```python
from build123d import *

# Parameters (mm, degrees)
SKETCH_W        = 100
SKETCH_H        = 84
PAD_DEPTH       = 10
SKETCH001_R     = 2.1
POCKET_DEPTH    = 10
SKETCH002_R     = 2.1
POCKET001_DEPTH = 10
SKETCH003_R     = 4
POCKET002_DEPTH = 4
SKETCH004_R     = 4
POCKET003_DEPTH = 4
SKETCH005_R     = 3.1
POCKET004_DEPTH = 10
SKETCH006_R     = 4.8
POCKET005_DEPTH = 5.2


with BuildPart() as part:
    # Sketch → Pad (new body)
    with BuildSketch(Plane.XY):
        with Locations((50, 42)):
            Rectangle(SKETCH_W, SKETCH_H)
    extrude(amount=PAD_DEPTH)

    # Sketch001 (on Face6 of Pad) → Pocket (cut)
    with BuildSketch(Plane.XY.offset(10)):
        with Locations((5, 6)):
            Circle(SKETCH001_R)
        with Locations((29, 6)):
            Circle(SKETCH001_R)
        with Locations((71, 6)):
            Circle(SKETCH001_R)
        with Locations((95, 6)):
            Circle(SKETCH001_R)
        with Locations((5, 24)):
            Circle(SKETCH001_R)
        with Locations((29, 24)):
            Circle(SKETCH001_R)
        with Locations((71, 24)):
            Circle(SKETCH001_R)
        with Locations((95, 24)):
            Circle(SKETCH001_R)
        with Locations((5, 78)):
            Circle(SKETCH001_R)
        with Locations((29, 78)):
            Circle(SKETCH001_R)
        with Locations((5, 60)):
            Circle(SKETCH001_R)
        with Locations((29, 60)):
            Circle(SKETCH001_R)
        with Locations((71, 78)):
            Circle(SKETCH001_R)
        with Locations((95, 78)):
            Circle(SKETCH001_R)
        with Locations((71, 60)):
            Circle(SKETCH001_R)
        with Locations((95, 60)):
            Circle(SKETCH001_R)
    extrude(amount=-POCKET_DEPTH, mode=Mode.SUBTRACT)

    # Sketch002 (on Face5 of Pocket) → Pocket001 (cut)
    with BuildSketch(Plane.XY.offset(10)):
        with Locations((35, 47)):
            Circle(SKETCH002_R)
        with Locations((65, 47)):
            Circle(SKETCH002_R)
        with Locations((35, 37)):
            Circle(SKETCH002_R)
        with Locations((65, 37)):
            Circle(SKETCH002_R)
    extrude(amount=-POCKET001_DEPTH, mode=Mode.SUBTRACT)

    # Sketch003 (on Face5 of Pocket001) → Pocket002 (cut)
    with BuildSketch(Plane.XY.offset(10)):
        with Locations((35, 47)):
            Circle(SKETCH003_R)
        with Locations((65, 47)):
            Circle(SKETCH003_R)
        with Locations((35, 37)):
            Circle(SKETCH003_R)
        with Locations((65, 37)):
            Circle(SKETCH003_R)
    extrude(amount=-POCKET002_DEPTH, mode=Mode.SUBTRACT)

    # Sketch004 (on Face5 of Pocket002) → Pocket003 (cut)
    with BuildSketch(Plane.XY.offset(10)):
        with Locations((5, 78)):
            Circle(SKETCH004_R)
        with Locations((29, 78)):
            Circle(SKETCH004_R)
        with Locations((5, 60)):
            Circle(SKETCH004_R)
        with Locations((29, 60)):
            Circle(SKETCH004_R)
        with Locations((5, 24)):
            Circle(SKETCH004_R)
        with Locations((29, 24)):
            Circle(SKETCH004_R)
        with Locations((5, 6)):
            Circle(SKETCH004_R)
        with Locations((29, 6)):
            Circle(SKETCH004_R)
        with Locations((71, 78)):
            Circle(SKETCH004_R)
        with Locations((71, 60)):
            Circle(SKETCH004_R)
        with Locations((95, 78)):
            Circle(SKETCH004_R)
        with Locations((95, 60)):
            Circle(SKETCH004_R)
        with Locations((71, 24)):
            Circle(SKETCH004_R)
        with Locations((95, 24)):
            Circle(SKETCH004_R)
        with Locations((71, 6)):
            Circle(SKETCH004_R)
        with Locations((95, 6)):
            Circle(SKETCH004_R)
    extrude(amount=-POCKET003_DEPTH, mode=Mode.SUBTRACT)

    # Sketch005 (on Face5 of Pocket003) → Pocket004 (cut)
    with BuildSketch(Plane.XY.offset(10)):
        with Locations((20, 62)):
            Circle(SKETCH005_R)
        with Locations((80, 62)):
            Circle(SKETCH005_R)
        with Locations((20, 22)):
            Circle(SKETCH005_R)
        with Locations((80, 22)):
            Circle(SKETCH005_R)
    extrude(amount=-POCKET004_DEPTH, mode=Mode.SUBTRACT)

    # Sketch006 (on Face4 of Pocket004) → Pocket005 (cut)
    with BuildSketch(Plane(origin=(0, 0, 0), x_dir=(1, 0, 0), z_dir=(0, 0, -1))):
        with Locations((20, -22)):
            Circle(SKETCH006_R)
        with Locations((20, -62)):
            Circle(SKETCH006_R)
        with Locations((80, -62)):
            Circle(SKETCH006_R)
        with Locations((80, -22)):
            Circle(SKETCH006_R)
    extrude(amount=-POCKET005_DEPTH, mode=Mode.SUBTRACT)


solid = part.part
```
Verification items for the finished model (mm, model axes). A direction names the side the tool comes from. Round coordinates to 2 decimals unless told otherwise and drop trailing zeros. Order: outer loops, then holes, each group sorted by start corner. A loop starts at its lowest first (then second) coordinate and runs counter-clockwise, first axis right, second up. Notation, with made-up numbers: (52.25, -32) -> (61.25, -32) arc R22 ccw to (61.25, -8) -> close; hole circle Ø2 at (16, 16.25). An arc over 180 degrees is marked (long way). Put each result on its own line as item: value. Start each with the question number.
(1) Section check B-B (y = 37). Enter the section's corners in (x, z), then the cut area to 3 significant figures.
(2) Section check A-A (x = 65). Enter the section's corners in (y, z).
(3) Material ranges on line 1 along Y through (x, z) = (80, 7); line 2 along Y through (x, z) = (35, 6.9); line 3 along Y through (x, z) = (29, 4.6), recorded low to high.
(4) Tool access check on faces 3 (the face through (6.13, 25.77, 3.04)), 4 (the face through (4.133, 2.095, 8.028)), 5 (the face through (15.205, 21.789, 2.564)). Record the directions out of +Z, -Z, +X, -X, +Y, -Y that give a thin tool (end or side, any length) a straight path to the whole face; none if there is none.
(5) Section check C-C (x = 5). State how many separate pieces and enclosed holes the cut face has, then the cut area to 3 significant figures.
(6) Depth check by flat-ended pin: pin 1 Ø5 at (x, y) = (29, 6) entering from +Z. Enter the tip coordinate at first touch or a pass-through.
(7) Draft check along X on faces 1 (the face through (92.9, 78.09, 3.04)), 2 (the face through (0, 41, 5)). Enter one of: +X half, -X half, draft (parallel to the pull), parting line (faces both ways), or undercut.
Completed:
1. outline: (0, 0) -> (32.9, 0) -> (32.9, 6) -> (31, 6) -> (31, 10) -> (0, 10) -> close; (37.1, 0) -> (62.9, 0) -> (62.9, 6) -> (61, 6) -> (61, 10) -> (39, 10) -> (39, 6) -> (37.1, 6) -> close; (67.1, 0) -> (100, 0) -> (100, 10) -> (69, 10) -> (69, 6) -> (67.1, 6) -> close
1. area: 886 mm2
2. outline: (0, 0) -> (34.9, 0) -> (34.9, 6) -> (33, 6) -> (33, 10) -> (0, 10) -> close; (39.1, 0) -> (44.9, 0) -> (44.9, 6) -> (43, 6) -> (43, 10) -> (41, 10) -> (41, 6) -> (39.1, 6) -> close; (49.1, 0) -> (84, 0) -> (84, 10) -> (51, 10) -> (51, 6) -> (49.1, 6) -> close
3. line 1: y = 0 to 18.9, 25.1 to 58.9, 65.1 to 84
3. line 2: y = 0 to 33, 41 to 43, 51 to 84
3. line 3: y = 0 to 3.9, 8.1 to 21.9, 26.1 to 57.9, 62.1 to 75.9, 80.1 to 84
4. face 3: +Z, -Z
4. face 4: +Z
4. face 5: -Z
5. separate pieces: 5
5. enclosed holes: 0
5. area: 611 mm2
6. pin 1: stops at z = 6
7. face 1: undercut
7. face 2: -X half
